Here's how the part is built. I have some questions about the finished solid (model axes, mm). Give positions to 0.01 mm unless a question says otherwise; leave off trailing zeros. Loops run counter-clockwise (first coordinate to the right, second up) from the corner with the lowest first, then second, coordinate; pieces in that order, holes last. Notation, with made-up numbers: (-20, -19.75) - (36, -19.75) arc R9 cw to (36, -15.75) - close; hole circle Ø4 at (81, 11.25). An arc over 180 degrees is marked (long way). Use a Markdown table: item, result.
from build123d import *

# Parameters (mm, degrees)
BOSS_EXTRUDE1_DEPTH = 6
CUT_EXTRUDE1_DEPTH  = 6


with BuildPart() as part:
    # Sketch1 → Boss-Extrude1 (new body)
    with BuildSketch(Plane.XY):
        with BuildLine():
            Line((20, 0), (260, 0))
            ThreePointArc((260, 0), (274.142135624, 5.857864376), (280, 20))
            Line((280, 20), (280, 140))
            ThreePointArc((280, 140), (274.142135624, 154.142135624), (260, 160))
            Line((260, 160), (20, 160))
            ThreePointArc((20, 160), (5.857864376, 154.142135624), (0, 140))
            Line((0, 140), (0, 20))
            ThreePointArc((0, 20), (5.857864376, 5.857864376), (20, 0))
        make_face()
    extrude(amount=BOSS_EXTRUDE1_DEPTH)

    # Sketch2 → Cut-Extrude1 (cut)
    with BuildSketch(Plane.XY.offset(6)):
        with BuildLine():
            Line((15, 137.5), (30, 137.5))
            Line((30, 137.5), (30, 120))
            ThreePointArc((30, 120), (31.153533726, 119.933245187), (32.291666667, 119.733871989))
            ThreePointArc((32.291666667, 119.733871989), (33.429799607, 119.933245187), (34.583333333, 120))
            Line((34.583333333, 120), (34.583333333, 137.5))
            Line((34.583333333, 137.5), (49.583333333, 137.5))
            Line((49.583333333, 137.5), (49.583333333, 120))
            ThreePointArc((49.583333333, 120), (50.736867059, 119.933245187), (51.875, 119.733871989))
            ThreePointArc((51.875, 119.733871989), (53.013132941, 119.933245187), (54.166666667, 120))
            Line((54.166666667, 120), (54.166666667, 137.5))
            Line((54.166666667, 137.5), (69.166666667, 137.5))
            Line((69.166666667, 137.5), (69.166666667, 120))
            ThreePointArc((69.166666667, 120), (70.320200393, 119.933245187), (71.458333333, 119.733871989))
            ThreePointArc((71.458333333, 119.733871989), (72.596466274, 119.933245187), (73.75, 120))
            Line((73.75, 120), (73.75, 137.5))
            Line((73.75, 137.5), (88.75, 137.5))
            Line((88.75, 137.5), (88.75, 120))
            ThreePointArc((88.75, 120), (89.903533726, 119.933245187), (91.041666667, 119.733871989))
            ThreePointArc((91.041666667, 119.733871989), (92.179799607, 119.933245187), (93.333333333, 120))
            Line((93.333333333, 120), (93.333333333, 137.5))
            Line((93.333333333, 137.5), (108.333333333, 137.5))
            Line((108.333333333, 137.5), (108.333333333, 120))
            ThreePointArc((108.333333333, 120), (109.486867059, 119.933245187), (110.625, 119.733871989))
            ThreePointArc((110.625, 119.733871989), (111.763132941, 119.933245187), (112.916666667, 120))
            Line((112.916666667, 120), (112.916666667, 137.5))
            Line((112.916666667, 137.5), (127.916666667, 137.5))
            Line((127.916666667, 137.5), (127.916666667, 120))
            ThreePointArc((127.916666667, 120), (129.070200393, 119.933245187), (130.208333333, 119.733871989))
            ThreePointArc((130.208333333, 119.733871989), (131.346466274, 119.933245187), (132.5, 120))
            Line((132.5, 120), (132.5, 137.5))
            Line((132.5, 137.5), (147.5, 137.5))
            Line((147.5, 137.5), (147.5, 120))
            ThreePointArc((147.5, 120), (148.653533726, 119.933245187), (149.791666667, 119.733871989))
            ThreePointArc((149.791666667, 119.733871989), (150.929799607, 119.933245187), (152.083333333, 120))
            Line((152.083333333, 120), (152.083333333, 137.5))
            Line((152.083333333, 137.5), (167.083333333, 137.5))
            Line((167.083333333, 137.5), (167.083333333, 120))
            ThreePointArc((167.083333333, 120), (168.236867059, 119.933245187), (169.375, 119.733871989))
            ThreePointArc((169.375, 119.733871989), (170.513132941, 119.933245187), (171.666666667, 120))
            Line((171.666666667, 120), (171.666666667, 137.5))
            Line((171.666666667, 137.5), (186.666666667, 137.5))
            Line((186.666666667, 137.5), (186.666666667, 120))
            ThreePointArc((186.666666667, 120), (187.820200393, 119.933245187), (188.958333333, 119.733871989))
            ThreePointArc((188.958333333, 119.733871989), (190.096466274, 119.933245187), (191.25, 120))
            Line((191.25, 120), (191.25, 137.5))
            Line((191.25, 137.5), (206.25, 137.5))
            Line((206.25, 137.5), (206.25, 120))
            ThreePointArc((206.25, 120), (207.403533726, 119.933245187), (208.541666667, 119.733871989))
            ThreePointArc((208.541666667, 119.733871989), (209.679799607, 119.933245187), (210.833333333, 120))
            Line((210.833333333, 120), (210.833333333, 137.5))
            Line((210.833333333, 137.5), (225.833333333, 137.5))
            Line((225.833333333, 137.5), (225.833333333, 120))
            ThreePointArc((225.833333333, 120), (226.986867059, 119.933245187), (228.125, 119.733871989))
            ThreePointArc((228.125, 119.733871989), (229.263132941, 119.933245187), (230.416666667, 120))
            Line((230.416666667, 120), (230.416666667, 137.5))
            Line((230.416666667, 137.5), (245.416666667, 137.5))
            Line((245.416666667, 137.5), (245.416666667, 120))
            ThreePointArc((245.416666667, 120), (246.570200393, 119.933245187), (247.708333333, 119.733871989))
            ThreePointArc((247.708333333, 119.733871989), (248.846466274, 119.933245187), (250, 120))
            Line((250, 120), (250, 137.5))
            Line((250, 137.5), (265, 137.5))
            Line((265, 137.5), (265, 120))
            ThreePointArc((265, 120), (275, 110), (265, 100))
            Line((265, 100), (265, 22.5))
            Line((265, 22.5), (250, 22.5))
            Line((250, 22.5), (250, 100))
            Line((250, 100), (245.416666667, 100))
            Line((245.416666667, 100), (245.416666667, 22.5))
            Line((245.416666667, 22.5), (230.416666667, 22.5))
            Line((230.416666667, 22.5), (230.416666667, 100))
            Line((230.416666667, 100), (225.833333333, 100))
            Line((225.833333333, 100), (225.833333333, 22.5))
            Line((225.833333333, 22.5), (210.833333333, 22.5))
            Line((210.833333333, 22.5), (210.833333333, 100))
            Line((210.833333333, 100), (206.25, 100))
            Line((206.25, 100), (206.25, 22.5))
            Line((206.25, 22.5), (191.25, 22.5))
            Line((191.25, 22.5), (191.25, 100))
            Line((191.25, 100), (186.666666667, 100))
            Line((186.666666667, 100), (186.666666667, 22.5))
            Line((186.666666667, 22.5), (171.666666667, 22.5))
            Line((171.666666667, 22.5), (171.666666667, 100))
            Line((171.666666667, 100), (167.083333333, 100))
            Line((167.083333333, 100), (167.083333333, 22.5))
            Line((167.083333333, 22.5), (152.083333333, 22.5))
            Line((152.083333333, 22.5), (152.083333333, 100))
            ThreePointArc((152.083333333, 100), (150.929799607, 100.066754813), (149.791666667, 100.266128011))
            ThreePointArc((149.791666667, 100.266128011), (148.653533726, 100.066754813), (147.5, 100))
            Line((147.5, 100), (147.5, 22.5))
            Line((147.5, 22.5), (132.5, 22.5))
            Line((132.5, 22.5), (132.5, 100))
            ThreePointArc((132.5, 100), (131.346466274, 100.066754813), (130.208333333, 100.266128011))
            ThreePointArc((130.208333333, 100.266128011), (129.070200393, 100.066754813), (127.916666667, 100))
            Line((127.916666667, 100), (127.916666667, 22.5))
            Line((127.916666667, 22.5), (112.916666667, 22.5))
            Line((112.916666667, 22.5), (112.916666667, 100))
            ThreePointArc((112.916666667, 100), (111.763132941, 100.066754813), (110.625, 100.266128011))
            ThreePointArc((110.625, 100.266128011), (109.486867059, 100.066754813), (108.333333333, 100))
            Line((108.333333333, 100), (108.333333333, 22.5))
            Line((108.333333333, 22.5), (93.333333333, 22.5))
            Line((93.333333333, 22.5), (93.333333333, 100))
            ThreePointArc((93.333333333, 100), (92.179799607, 100.066754813), (91.041666667, 100.266128011))
            ThreePointArc((91.041666667, 100.266128011), (89.903533726, 100.066754813), (88.75, 100))
            Line((88.75, 100), (88.75, 22.5))
            Line((88.75, 22.5), (73.75, 22.5))
            Line((73.75, 22.5), (73.75, 100))
            ThreePointArc((73.75, 100), (72.596466274, 100.066754813), (71.458333333, 100.266128011))
            ThreePointArc((71.458333333, 100.266128011), (70.320200393, 100.066754813), (69.166666667, 100))
            Line((69.166666667, 100), (69.166666667, 22.5))
            Line((69.166666667, 22.5), (54.166666667, 22.5))
            Line((54.166666667, 22.5), (54.166666667, 100))
            ThreePointArc((54.166666667, 100), (53.013132941, 100.066754813), (51.875, 100.266128011))
            ThreePointArc((51.875, 100.266128011), (50.736867059, 100.066754813), (49.583333333, 100))
            Line((49.583333333, 100), (49.583333333, 22.5))
            Line((49.583333333, 22.5), (34.583333333, 22.5))
            Line((34.583333333, 22.5), (34.583333333, 100))
            ThreePointArc((34.583333333, 100), (33.429799607, 100.066754813), (32.291666667, 100.266128011))
            ThreePointArc((32.291666667, 100.266128011), (31.153533726, 100.066754813), (30, 100))
            Line((30, 100), (30, 22.5))
            Line((30, 22.5), (15, 22.5))
            Line((15, 22.5), (15, 100))
            ThreePointArc((15, 100), (5, 110), (15, 120))
            Line((15, 120), (15, 137.5))
        make_face()
    extrude(amount=-CUT_EXTRUDE1_DEPTH, mode=Mode.SUBTRACT)


solid = part.part
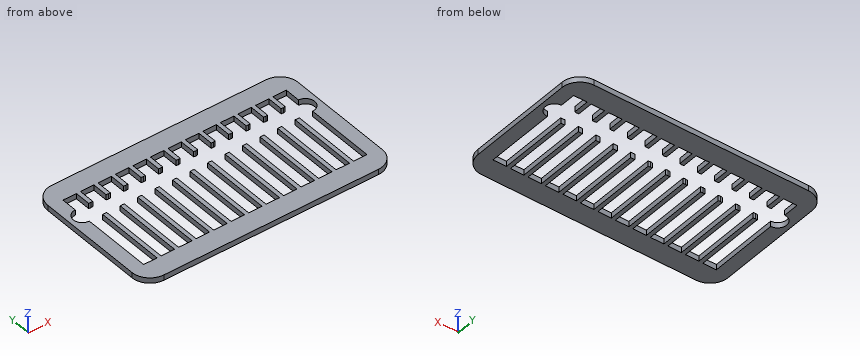
(1) Will this pin go through, and if not, where does the flat tip stop? pin 1 (6 mm diameter, centred on x = 168.5, y = 104.5, fed in from -Z).
A:
| item | result |
|---|---|
| pin 1 | through |
(2) If I drill on line 1 (Y direction, x = 49, z = 5.45); line 2 (Y direction, x = 150, z = 1.6); line 3 (X direction, y = 16.5, z = 0.3), over which ranges is the centre line in solid material (lowest first)?
A:
| item | result |
|---|---|
| line 1 | 0 to 22.5, 137.5 to 160 |
| line 2 | 0 to 100.22, 119.78 to 160 |
| line 3 | 0.31 to 279.69 |
(3) Suppose I cut it at A-A on y = 110. Write out the boundary of the cut face in (x, z), plus the area to 3 significant figures.
A:
| item | result |
|---|---|
| outline | (0, 0) - (5, 0) - (5, 6) - (0, 6) - close; (275, 0) - (280, 0) - (280, 6) - (275, 6) - close |
| area | 60.0 mm2 |
(4) Suppose I cut it at B-B on y = 68.5. Count the separate pieces of the cut face and the enclosed holes in it, plus the area to 3 significant figures.
A:
| item | result |
|---|---|
| separate pieces | 14 |
| enclosed holes | 0 |
| area | 510 mm2 |
